Study the drawing (mm; zero at the part's minimum x, y, z) and answer. Coordinates: 2 decimals unless noted, no trailing zeros. Loops run counter-clockwise (first coordinate to the right, second up) from the corner with the lowest first, then second, coordinate; pieces in that order, holes last.
Q1. Section D-D (y = 30) is taken. Give the vertices of the cut face in (x, z).
Q2. Flat-ended cylindrical pins translate along their axes: P1, Ø6, axis at x = 7.5, z = 27.5, coming from the -Y side; P2, Ø3, axis at x = 4.5, z = 53, coming from the +Y side; P3, Ø1, axis at x = 2.5, z = 56.5, coming from the -Y side. Find the tip coordinate at first contact, or state that the pin passes through.
Q3. Section C-C (y = 55) is taken. Give the vertices of the cut face in (x, z).
Q4. Section A-A (z = 55) is taken. Give the vertices of the cut face in (x, y).
Q5. Straight lines are drawn through the part: line 1 (Y direction, x = 4, z = 55); line 2 (Z direction, x = 6.5, y = 30); line 3 (Y direction, x = 4, z = 56). For each, find the intervals that lie inside material, in ascending order.
Q6. The mould has two halves that part along Z. Classify the marked faces 1 and 2: pulls with the +Z half, pulls with the -Z half, needs draft (parallel to the pull), parting line crosses it, or undercut.
Q7. Section B-B (x = 2.5) is taken. Give the vertices of the cut face in (y, z).
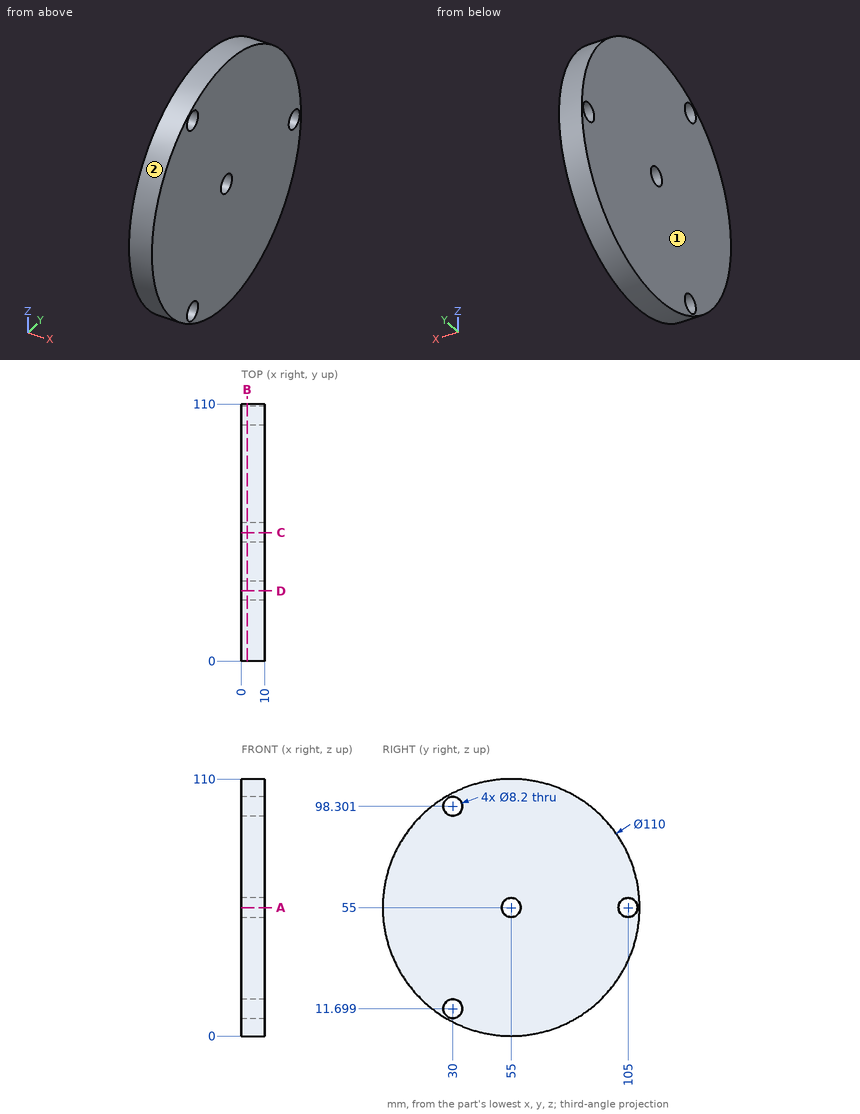
Numbers:
1. outline: (0, 6.01) - (10, 6.01) - (10, 7.6) - (0, 7.6) - close; (0, 15.8) - (10, 15.8) - (10, 94.2) - (0, 94.2) - close; (0, 102.4) - (10, 102.4) - (10, 103.99) - (0, 103.99) - close
2. P1: stops at y = 5.76
2. P2: stops at y = 110
2. P3: stops at y = 0.01
3. outline: (0, 0) - (10, 0) - (10, 50.9) - (0, 50.9) - close; (0, 59.1) - (10, 59.1) - (10, 110) - (0, 110) - close
4. outline: (0, 0) - (10, 0) - (10, 50.9) - (0, 50.9) - close; (0, 59.1) - (10, 59.1) - (10, 100.9) - (0, 100.9) - close; (0, 109.1) - (10, 109.1) - (10, 110) - (0, 110) - close
5. line 1: y = 0 to 50.9, 59.1 to 100.9, 109.1 to 110
5. line 2: z = 6.01 to 7.6, 15.8 to 94.2, 102.4 to 103.99
5. line 3: y = 0.01 to 51.02, 58.98 to 101.02, 108.98 to 109.99
6. face 1: needs draft
6. face 2: parting line crosses it
7. outline: circle Ø110 at (55, 55); hole circle Ø8.2 at (30, 11.7); hole circle Ø8.2 at (30, 98.3); hole circle Ø8.2 at (55, 55); hole circle Ø8.2 at (105, 55)
